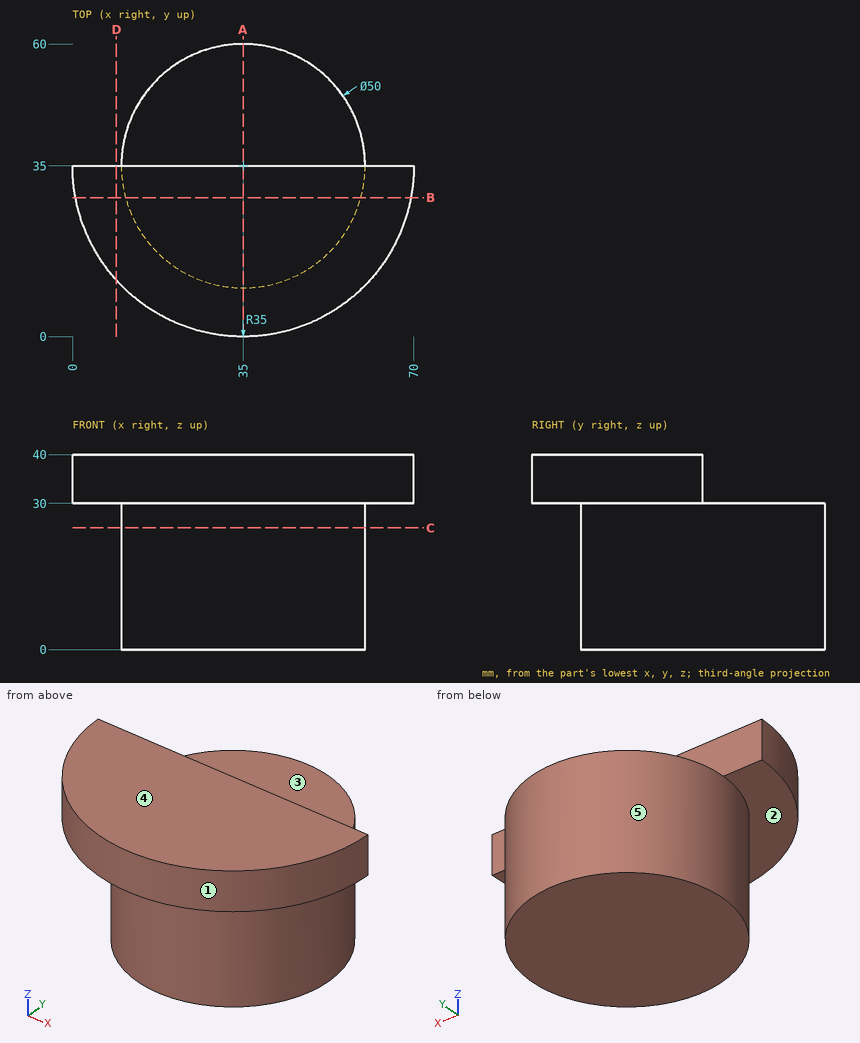
Geometry check sheet. Reference: drawing and pictorial views, mm from the part's lowest x, y, z. A direction names the side the tool comes from. Round coordinates to 2 decimals unless told otherwise and drop trailing zeros. Loops run counter-clockwise (first coordinate to the right, second up) from the corner with the lowest first, then second, coordinate; pieces in that order, holes last. Notation, with made-up numbers: (44.5, -14) -> (88.5, -14) arc R24 cw to (88.5, 22) -> close; hole circle Ø9 at (59.5, 54.5). An arc over 180 degrees is marked (long way). Answer as a JSON object with one key per item and string values. Group by question number.
Item 1: Thickness scan on line 1 along Z through (x, y) = (52, 14); line 2 along Z through (x, y) = (31.5, 47); line 3 along Y through (x, z) = (12.5, 22). Record the ranges inside material, lowest first.
Item 2: Cross-section at D-D, the plane x = 9. Record the cut outline in (y, z), plus the area to 3 significant figures.
Item 3: Cross-section at B-B, the plane y = 28.5. Record the cut outline in (x, z), plus the area to 3 significant figures.
Item 4: Cross-section at A-A, the plane x = 35. Record the cut outline in (y, z), plus the area to 3 significant figures.
Item 5: Set-up check for the marked faces 1, 2, 3, 4 and 5: record each of +Z, -Z, +X, -X, +Y, -Y from which the full face is reachable in a straight line by a thin tool's end or side.
Item 6: Cross-section at C-C, the plane z = 25. Record the cut outline in (x, y).
Item 7: Depth check by flat-ended pin: pin 1 Ø3 at (x, z) = (62, 27.5) entering from -Y; pin 2 Ø1 at (x, z) = (39.5, 21) entering from -Y; pin 3 Ø5 at (x, z) = (45.5, 17) entering from +Y; pin 4 Ø5 at (x, z) = (60.5, 11) entering from -Y. Enter the tip coordinate at first touch or a pass-through.
Determined:
{
 "1": {"line 1": "z = 30 to 40", "line 2": "z = 0 to 30", "line 3": "y = 24.1 to 45.9"},
 "2": {"outline": "(11.57, 30) -> (35, 30) -> (35, 40) -> (11.57, 40) -> close", "area": "234 mm²"},
 "3": {"outline": "(0.61, 30) -> (10.86, 30) -> (10.86, 0) -> (59.14, 0) -> (59.14, 30) -> (69.39, 30) -> (69.39, 40) -> (0.61, 40) -> close", "area": "2,140 mm²"},
 "4": {"outline": "(0, 30) -> (10, 30) -> (10, 0) -> (60, 0) -> (60, 30) -> (35, 30) -> (35, 40) -> (0, 40) -> close", "area": "1,850 mm²"},
 "5": {"face 1": "+Z, -Z, -Y", "face 2": "-Z, -Y", "face 3": "+Z, +X, -X, +Y", "face 4": "+Z, +X, -X, +Y, -Y", "face 5": "-Z"},
 "6": {"outline": "circle Ø50 at (35, 35)"},
 "7": {"pin 1": "passes through", "pin 2": "stops at y = 10.32", "pin 3": "stops at y = 58.69", "pin 4": "stops at y = 25.2"}
}
